The listing builds one solid part. Answer for the finished solid, in the listing's coordinates (mm). Face numbers are marked on the shaded views. A direction names the side the tool comes from. Round coordinates to 2 decimals unless told otherwise and drop trailing zeros. Loops run counter-clockwise (first coordinate to the right, second up) from the corner with the lowest first, then second, coordinate; pieces in that order, holes last. Notation, with made-up numbers: (27.5, 52.5) -> (42.5, 52.5) arc R14 ccw to (42.5, 64.5) -> close; hole circle Ø10 at (-15.5, 10). An arc over 180 degrees is marked (long way). Use a Markdown table: item, result. Add a question column.
Q1. Which of the six approach directions +Z, -Z, +X, -X, +Y, -Y give full straight-line access (tool end or side, diameter ignored) to the marked faces 1, 2 and 3?
Q2. Section A-A on y = 0 is taken. Give the vertices of the cut face in (x, z), then the cut area to 3 significant figures.
Q3. For a pull along X with two mould halves and no side action, classify the marked faces 4, 5, 6 and 7 as released by +X, released by -X, zero draft, split by the parting line, or undercut.
Q4. Consider line 1 (Z direction, x = -1.5, y = -3.75); line 2 (Z direction, x = 3, y = -7); line 3 (Y direction, x = -5.5, z = 26). Determine where each line is inside the solid, lowest interval first.
Q5. Section C-C on x = 0 is taken. Give the vertices of the cut face in (y, z).
Q6. Given pin 1 Ø5 at (y, z) = (-2.5, 27) entering from -X; pin 2 Ø4 at (y, z) = (-5, 23.5) entering from +X; pin 3 Ø8 at (x, z) = (5, 10) entering from -Y, each flat-ended and moving along its own axis, determine where each tip first touches the part or whether it passes through.
Q7. Section D-D on z = 26 is taken. Give the vertices of the cut face in (x, y), then the cut area to 3 significant figures.
Q8. Section B-B on z = 21 is taken. Give the vertices of the cut face in (x, y).
from build123d import *

# Parameters (mm, degrees)
SKETCH1_R               = 7.5
BOSS_EXTRUDE1_DEPTH     = 30
SKETCH3_W               = 10
SKETCH3_H               = 16
CUT_EXTRUDE2_DEPTH      = 10
CUT_EXTRUDE3_DEPTH      = 32.819805153
CUT_EXTRUDE3_DEPTH_BACK = 32.819805153
CUT_EXTRUDE4_DEPTH      = 32.819805295
CUT_EXTRUDE4_DEPTH_BACK = 32.819805295
SKETCH5_R               = 1.5
FILLET1_R               = 0.1
SKETCH6_W               = 20
SKETCH6_H               = 20
BOSS_EXTRUDE2_DEPTH     = 3


with BuildPart() as part:
    # Sketch1 → Boss-Extrude1 (new body)
    with BuildSketch(Plane.XY):
        Circle(SKETCH1_R)
    extrude(amount=BOSS_EXTRUDE1_DEPTH)

    # Sketch3 → Cut-Extrude2 (cut)
    with BuildSketch(Plane.XY.offset(30)):
        Rectangle(SKETCH3_W, SKETCH3_H)
    extrude(amount=-CUT_EXTRUDE2_DEPTH, mode=Mode.SUBTRACT)

    # Sketch4 → Cut-Extrude3 (cut, two sides: drawn at the far end of the back side and taken through both)
    with BuildSketch(Plane(origin=(0, 0, 0), x_dir=(0, 0, -1), z_dir=(1, 0, 0)).offset(-CUT_EXTRUDE3_DEPTH_BACK)):
        with BuildLine():
            Line((-20, 67.5), (-20, 7.5))
            Line((-20, 7.5), (-20, 5.590169944))
            Line((-20, 5.590169944), (-26.952923855, 3.884664175))
            ThreePointArc((-26.952923855, 3.884664175), (-29.999999999, -0.000262165), (-26.952744721, -3.885047998))
            Line((-26.952744721, -3.885047998), (-20, -5.590169944))
            Line((-20, -5.590169944), (-20, -7.5))
            Line((-20, -7.5), (-20, -67.5))
            Line((-20, -67.5), (-140, -67.5))
            Line((-140, -67.5), (-140, 67.5))
            Line((-140, 67.5), (-20, 67.5))
        make_face()
    extrude(amount=CUT_EXTRUDE3_DEPTH + CUT_EXTRUDE3_DEPTH_BACK, mode=Mode.SUBTRACT)

    # Sketch5 → Cut-Extrude4 (cut, two sides: drawn at the far end of the back side and taken through both)
    with BuildSketch(Plane(origin=(0, 0, 0), x_dir=(0, 0, -1), z_dir=(1, 0, 0)).offset(-CUT_EXTRUDE4_DEPTH_BACK)):
        with Locations(Location((-26, -0.000169944, 0), (0, 0, 0.006491373))):
            Circle(SKETCH5_R)
    extrude(amount=CUT_EXTRUDE4_DEPTH + CUT_EXTRUDE4_DEPTH_BACK, mode=Mode.SUBTRACT)

    # Fillet1
    # the kernel refuses this fillet: 0.1 mm, written as the material it takes off along each edge
    with BuildSketch(Plane(origin=(0, 0, 20), x_dir=(0.6911452834399253, -0.7227158481580055, 0), z_dir=(0.7227158481580055, 0.6911452834399253, 0))) as fillet1_piece_1_section:
        with BuildLine():
            CenterArc((7.5 - FILLET1_R, FILLET1_R), FILLET1_R, 270, 90)
            Line((7.5 - FILLET1_R, 0), (7.5, 0))
            Line((7.5, 0), (7.5, FILLET1_R))
        make_face()
    fillet1_piece_1 = revolve(axis=Axis((0, 0, 20), (0, 0, -1)), revolution_arc=87.441672972, mode=Mode.PRIVATE)
    fillet1_piece_1 = split(fillet1_piece_1, bisect_by=Plane(origin=(5, -5.569278589, 19.983070115), z_dir=(-1, 0, 0)), keep=Keep.TOP, mode=Mode.PRIVATE)
    fillet1_piece_1 = split(fillet1_piece_1, bisect_by=Plane(origin=(-5, -5.569278589, 19.983070115), z_dir=(1, 0, 0)), keep=Keep.TOP, mode=Mode.PRIVATE)
    add(fillet1_piece_1, mode=Mode.SUBTRACT)
    with BuildSketch(Plane(origin=(0, 0, 20), x_dir=(-0.6911452834399255, 0.7227158481580054, 0), z_dir=(-0.7227158481580054, -0.6911452834399255, 0))) as fillet1_piece_2_section:
        with BuildLine():
            CenterArc((7.5 - FILLET1_R, FILLET1_R), FILLET1_R, 270, 90)
            Line((7.5 - FILLET1_R, 0), (7.5, 0))
            Line((7.5, 0), (7.5, FILLET1_R))
        make_face()
    fillet1_piece_2 = revolve(axis=Axis((0, 0, 20), (0, 0, -1)), revolution_arc=87.441672972, mode=Mode.PRIVATE)
    fillet1_piece_2 = split(fillet1_piece_2, bisect_by=Plane(origin=(5, 5.569279486, 19.983069507), z_dir=(-1, 0, 0)), keep=Keep.TOP, mode=Mode.PRIVATE)
    fillet1_piece_2 = split(fillet1_piece_2, bisect_by=Plane(origin=(-5, 5.569279486, 19.983069507), z_dir=(1, 0, 0)), keep=Keep.TOP, mode=Mode.PRIVATE)
    add(fillet1_piece_2, mode=Mode.SUBTRACT)

    # Sketch6 → Boss-Extrude2 (add)
    with BuildSketch(Plane(origin=(0, 0, 0), x_dir=(-1, 0, 0), z_dir=(0, 0, -1))):
        Rectangle(SKETCH6_W, SKETCH6_H)
    extrude(amount=BOSS_EXTRUDE2_DEPTH)


solid = part.part
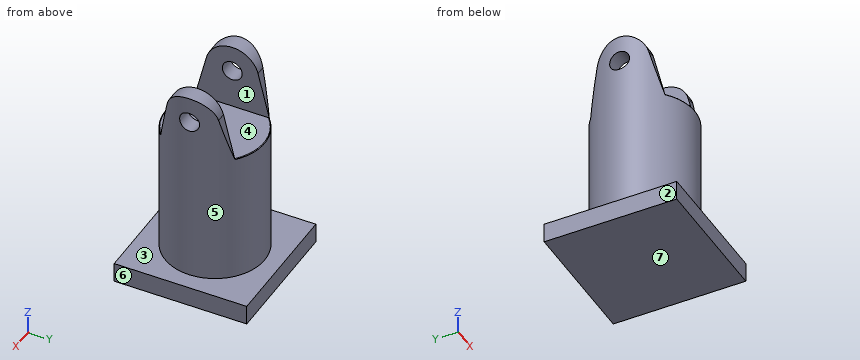
Checked values:
| question | item | result |
|---|---|---|
| 1 | face 1 | +Z, +Y, -Y |
| 1 | face 2 | +Z, -Z, -X, +Y, -Y |
| 1 | face 3 | +Z |
| 2 | outline | (-10, -3) -> (10, -3) -> (10, 0) -> (7.5, 0) -> (7.5, 24.5) -> (5, 24.5) -> (5, 20) -> (-5, 20) -> (-5, 24.5) -> (-7.5, 24.5) -> (-7.5, 0) -> (-10, 0) -> close; (-7.5, 27.5) -> (-5, 27.5) -> (-5, 30) -> (-7.5, 30) -> close; (5, 27.5) -> (7.5, 27.5) -> (7.5, 30) -> (5, 30) -> close |
| 2 | area | 395 mm2 |
| 3 | face 4 | undercut |
| 3 | face 5 | split by the parting line |
| 3 | face 6 | released by +X |
| 3 | face 7 | zero draft |
| 4 | line 1 | z = -3 to 20 |
| 4 | line 2 | z = -3 to 0 |
| 4 | line 3 | y = -4.12 to -1.5, 1.5 to 4.12 |
| 5 | outline | (-10, -3) -> (10, -3) -> (10, 0) -> (7.5, 0) -> (7.5, 19.9) arc R0.1 ccw to (7.4, 20) -> (-7.4, 20) arc R0.1 ccw to (-7.5, 19.9) -> (-7.5, 0) -> (-10, 0) -> close |
| 6 | pin 1 | stops at x = -7.5 |
| 6 | pin 2 | stops at x = 6.87 |
| 6 | pin 3 | stops at y = -7.43 |
| 7 | outline | (-7.35, -1.5) arc R7.5 ccw to (-6.27, -4.12) -> (-5, -4.12) -> (-5, -1.5) -> close; (-7.35, 1.5) -> (-5, 1.5) -> (-5, 4.12) -> (-6.27, 4.12) arc R7.5 ccw to start; (5, -4.12) -> (6.27, -4.12) arc R7.5 ccw to (7.35, -1.5) -> (5, -1.5) -> close; (5, 1.5) -> (7.35, 1.5) arc R7.5 ccw to (6.27, 4.12) -> (5, 4.12) -> close |
| 7 | area | 20.0 mm2 |
| 8 | outline | (-5.26, -5.34) -> (-5, -5.34) -> (-5, 5.34) -> (-5.26, 5.34) arc R7.5 ccw to start; (5, -5.34) -> (5.26, -5.34) arc R7.5 ccw to (5.26, 5.34) -> (5, 5.34) -> close |
